Verification items for the finished model (mm, model axes). Face numbers are marked on the shaded views. A direction names the side the tool comes from. Round coordinates to 2 decimals unless told otherwise and drop trailing zeros. Loops run counter-clockwise (first coordinate to the right, second up) from the corner with the lowest first, then second, coordinate; pieces in that order, holes last. Notation, with made-up numbers: (25.5, 69) - (54.5, 69) arc R17 cw to (54.5, 95) - close; hole circle Ø9 at (43, -35.5). An arc over 180 degrees is marked (long way). Use a Markdown table: item, result. Add a question column.
```python
from build123d import *

# Parameters (mm, degrees)
BOSS_EXTRUDE1_DEPTH = 10
SKETCH3_R           = 1.5
CUT_EXTRUDE1_DEPTH  = 74.703487344
SKETCH5_R           = 10
CUT_EXTRUDE2_DEPTH  = 10
CIRPATTERN1_COUNT   = 3


with BuildPart() as part:
    # Sketch1 → Boss-Extrude1 (new body)
    with BuildSketch(Plane.XY):
        Polygon((-36.510971114, 21.079619001), (-26.510971114, 21.079619001), (-26.510971114, -21.079619001), (-36.510971114, -21.079619001), (0, -42.159238002), (-5, -33.498983964), (31.510971114, -12.419364963), (36.510971114, -21.079619001), (36.510971114, 21.079619001), (31.510971114, 12.419364963), (-5, 33.498983964), (0, 42.159238002), align=None)
    extrude(amount=BOSS_EXTRUDE1_DEPTH)

    # Sketch3 → Cut-Extrude1 (cut, symmetric)
    with BuildSketch(Plane(origin=(0, -21.079619001, 0), x_dir=(1, 0, 0), z_dir=(0, 1, 0))):
        with Locations(Location((-33.010971114, -5, 0), (0, 0, 90))):
            Circle(SKETCH3_R)
    cut_extrude1 = extrude(amount=CUT_EXTRUDE1_DEPTH, both=True, mode=Mode.SUBTRACT)

    # Sketch5 → Cut-Extrude2 (cut)
    with BuildSketch(Plane(origin=(0, 0, 0), x_dir=(-1, 0, 0), z_dir=(0, 0, -1))):
        Circle(SKETCH5_R)
    extrude(amount=-CUT_EXTRUDE2_DEPTH, mode=Mode.SUBTRACT)

    # CirPattern1: Cut-Extrude1 ×3 about axis
    cirpattern1_axis = Axis((0, 0, 10), (0, 0, -1))
    for i in range(1, CIRPATTERN1_COUNT):
        add(cut_extrude1.rotate(cirpattern1_axis, i * 360 / CIRPATTERN1_COUNT), mode=Mode.SUBTRACT)


solid = part.part
```
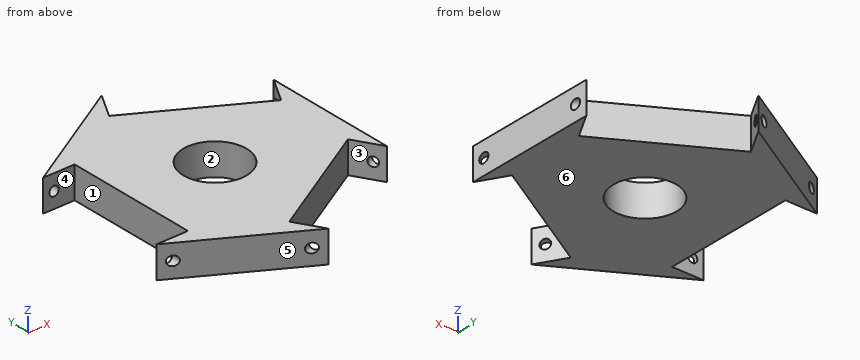
Q1. Set-up check for the marked faces 1, 2 and 3: record each of +Z, -Z, +X, -X, +Y, -Y from which the full face is reachable in a straight line by a thin tool's end or side.
Q2. Section check B-B on z = 2.25. Record the cut outline in (x, y), plus the area to 3 significant figures.
Q3. Section check C-C on x = -7. Record the cut outline in (y, z).
Q4. Go/stop test with flat-tipped pins: pin 1 Ø3 at (y, z) = (-9, 2.5) entering from -X; pin 2 Ø1 at (x, z) = (-6.5, 5) entering from +Y; pin 3 Ø3.5 at (x, z) = (-33.01, 5) entering from +Y. Record where each tip stops, or that it passes through.
Q5. Section check A-A on y = 0. Record the cut outline in (x, z), plus the area to 3 significant figures.
Q6. Release check for a two-part mould opening along Y. For the marked faces 4, 5 and 6 record: +Y half, -Y half, draft (parallel to the pull), parting line (faces both ways), or undercut.
Q7. Section check D-D on x = -21. Record the cut outline in (y, z).
Q8. Thickness scan on line 1 along Y through (x, z) = (-6, 4); line 2 along Y through (x, z) = (-0.5, 6.5); line 3 along X through (y, z) = (-7, 2.5). Record the ranges inside material, lowest first.
Determined:
| question | item | result |
|---|---|---|
| 1 | face 1 | +Z, -Z, -X |
| 1 | face 2 | +Z, -Z |
| 1 | face 3 | +Z, -Z, -Y |
| 2 | outline | (-36.51, -21.08) - (0, -42.16) - (-5, -33.5) - (31.51, -12.42) - (36.51, -21.08) - (36.51, 21.08) - (31.51, 12.42) - (-5, 33.5) - (0, 42.16) - (-36.51, 21.08) - (-26.51, 21.08) - (-26.51, -21.08) - close; hole circle Ø20 at (0, 0) |
| 2 | area | 3,040 mm² |
| 3 | outline | (-38.12, 0) - (-7.14, 0) - (-7.14, 10) - (-38.12, 10) - close; (7.14, 0) - (38.12, 0) - (38.12, 10) - (7.14, 10) - close |
| 4 | pin 1 | stops at x = -26.51 |
| 4 | pin 2 | stops at y = 38.7 |
| 4 | pin 3 | stops at y = 24.11 |
| 5 | outline | (-26.51, 0) - (-10, 0) - (-10, 10) - (-26.51, 10) - close; (10, 0) - (36.51, 0) - (36.51, 10) - (10, 10) - close |
| 5 | area | 430 mm² |
| 6 | face 4 | undercut |
| 6 | face 5 | -Y half |
| 6 | face 6 | draft |
| 7 | outline | (-30.03, 0) - (30.03, 0) - (30.03, 10) - (-30.03, 10) - close |
| 8 | line 1 | y = -38.7 to -8, 8 to 38.7 |
| 8 | line 2 | y = -41.87 to -41.29, -30.9 to -9.99, 9.99 to 30.9, 41.29 to 41.87 |
| 8 | line 3 | x = -26.51 to -7.14, 7.14 to 36.51 |
